from build123d import *

# Parameters (mm, degrees)
F0_W     = 203.2
F0_H     = 127
F1_DEPTH = 127
F3_DEPTH = 101.6
F4_SIZE2 = 101.6
F4_SIZE  = 76.2
F5_R     = 5.08


with BuildPart() as f1:
    # F0 (on Front) → F1 (new body)
    with BuildSketch(Plane.XZ):
        with Locations((-38.8936437666, -15.1942830797)):
            Rectangle(F0_W, F0_H)
    extrude(amount=F1_DEPTH)

    # F2 (on face) → F3 (cut)
    with BuildSketch(Plane.XZ.offset(127)):
        Polygon((62.7063562334, 48.3057169203), (-55.4564334452, 48.3057169203), (-55.4564334452, 0), (-85.3614583611, 0), (-85.3614583611, -78.6942830797), (62.7063562334, -78.6942830797), align=None)
    extrude(amount=-F3_DEPTH, mode=Mode.SUBTRACT)

    # F4
    f4_edges = [f1.edges().sort_by_distance(p)[0] for p in [
        (62.706356, -12.7, 48.305717),
    ]]
    f4_side = f1.faces().sort_by_distance((-75.879953, -52.452457, 48.305717))[0]
    chamfer(f4_edges, length=F4_SIZE, length2=F4_SIZE2, reference=f4_side)

    # F5
    f5_edges = [f1.edges().sort_by_distance(p)[0] for p in [
        (-55.456433, -76.2, 48.305717),
        (-34.475039, -25.4, 48.305717),
        (-13.493644, -12.7, 48.305717),
        (62.706356, -12.7, -53.294283),
        (24.606356, -25.4, -2.494283),
        (24.606356, 0, -2.494283),
        (62.706356, -25.4, -65.994283),
        (62.706356, -12.7, -78.694283),
        (62.706356, 0, -65.994283),
        (-55.456433, -25.4, 24.152858),
        (-70.408946, -25.4, 0),
        (-11.327551, -25.4, -78.694283),
        (-85.361458, -25.4, -39.347142),
        (-85.361458, -76.2, 0),
        (-85.361458, -76.2, -78.694283),
        (-85.361458, -127, -39.347142),
        (-97.975039, -127, 48.305717),
        (-55.456433, -127, 24.152858),
        (-70.408946, -127, 0),
        (-112.927551, -127, -78.694283),
        (-140.493644, -127, -15.194283),
        (-76.993644, 0, 48.305717),
        (-140.493644, -63.5, 48.305717),
    ]]
    fillet(f5_edges, radius=F5_R)


solid = f1.part
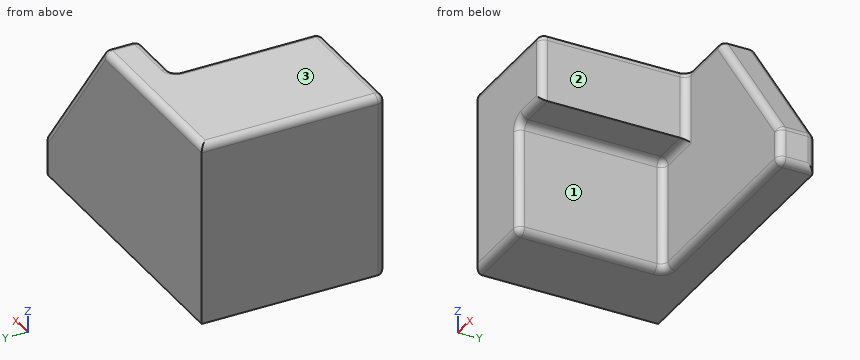
Build history of the part. All positions in model axes, mm. Face numbers are marked on the shaded views. A direction names the side the tool comes from. Give positions to 0.01 mm unless a question says otherwise; leave off trailing zeros. Loops run counter-clockwise (first coordinate to the right, second up) from the corner with the lowest first, then second, coordinate; pieces in that order, holes last. Notation, with made-up numbers: (27.5, 7) - (86.5, 7) arc R35 cw to (86.5, 46) - close; hole circle Ø11 at (80, -4.75). An arc over 180 degrees is marked (long way). Write item = value, one per line. Start each with the question number.
1) Drop flat-ended pins along their axis: pin 1 Ø20 at (x, y) = (-71, -72.5) entering from -Z; pin 2 Ø2 at (x, z) = (-58, -54.5) entering from +Y; pin 3 Ø4 at (x, z) = (-37.5, -7.5) entering from -Y; pin 4 Ø8 at (x, y) = (-84.5, -33.5) entering from -Z. Give the stop position or say it passes through.
2) Band-saw the part on A-A on y = -102.5. Give the cut face in (x, z), plus the area to 3 significant figures.
3) Tool access for the marked faces 1, 2 and 3: list every direction of +Z, -Z, +X, -X, +Y, -Y with a clear straight run to the whole face (end or side of a thin tool).
4) Probe probe 1 along X at (y, z) = (-108, 37); probe 2 along X at (y, z) = (-113.5, -36); probe 3 along Y at (x, z) = (21.5, -62). List the from-to ranges inside material, lowest first. Write a range as from..to.
5) Band-saw the part on B-B on z = -58.5. Give the cut face in (x, y).
Final values:
q1.pin_1 = -0.05
q1.pin_2 = 0
q1.pin_3 = -25.4
q1.pin_4 = -78.31
q2.outline = (-140.49, -78.69) - (-90.44, -78.69) arc R5.08 ccw to (-85.36, -73.61) - (-85.36, -5.08) arc R5.08 cw to (-80.28, 0) - (-55.46, 0) - (-55.46, 43.23) arc R5.08 ccw to (-60.54, 48.31) - (-135.41, 48.31) arc R5.08 ccw to (-140.49, 43.23) - close
q2.area = 8,440 mm²
q3.face_1 = -Z, +X, -Y
q3.face_2 = +Z, -Z, +X, -Y
q3.face_3 = +Z, +X, -X, +Y, -Y
q4.probe_1 = -140.49..-55.46
q4.probe_2 = -140.49..-85.36
q4.probe_3 = -25.4..0
q5.outline = (-140.49, -121.92) arc R5.08 ccw to (-135.41, -127) - (-90.44, -127) arc R5.08 ccw to (-85.36, -121.92) - (-85.36, -30.48) arc R5.08 cw to (-80.28, -25.4) - (57.63, -25.4) arc R5.08 ccw to (62.71, -20.32) - (62.71, -5.08) arc R5.08 ccw to (57.63, 0) - (-140.49, 0) - close
